```python
from build123d import *

# Parameters (mm, degrees)
SKETCH1_W          = 76
SKETCH1_H          = 76
SKETCH1_R          = 2
SKETCH1_R_2        = 16.65
BASE_FLANGE1_DEPTH = 1.6


# Sheet-metal steps are written as plain solids
with BuildPart() as part:
    # Sketch1 → Base-Flange1 (new body)
    with BuildSketch(Plane(origin=(0, 0, 0), x_dir=(1, 0, 0), z_dir=(0, 1, 0))):
        Rectangle(SKETCH1_W, SKETCH1_H)
        with Locations(Location((32.55, 32.55, 0), (0, 0, 270))):
            Circle(SKETCH1_R, mode=Mode.SUBTRACT)
        with Locations(Location((0, 0, 0), (0, 0, 270))):
            Circle(SKETCH1_R_2, mode=Mode.SUBTRACT)
        with Locations(Location((32.55, -32.55, 0), (0, 0, 270))):
            Circle(SKETCH1_R, mode=Mode.SUBTRACT)
        with Locations(Location((-32.55, -32.55, 0), (0, 0, 270))):
            Circle(SKETCH1_R, mode=Mode.SUBTRACT)
        with Locations(Location((-32.55, 32.55, 0), (0, 0, 270))):
            Circle(SKETCH1_R, mode=Mode.SUBTRACT)
    extrude(amount=-BASE_FLANGE1_DEPTH)


solid = part.part
```
Could you check a few things on this model? Use its own coordinates, in mm. Round coordinates to 2 decimals unless told otherwise and drop trailing zeros. Loops run counter-clockwise (first coordinate to the right, second up) from the corner with the lowest first, then second, coordinate; pieces in that order, holes last. Notation, with made-up numbers: (-28, -17.5) -> (-21, -17.5) arc R24 ccw to (-21, 12.5) -> close; hole circle Ø7 at (58, -9). An arc over 180 degrees is marked (long way). One line per question, with ' | ' between items.
(1) For pin 1 Ø5 at (x, z) = (-32.55, 32.55) entering from +Y; pin 2 Ø3.5 at (x, z) = (32.55, -32.55) entering from -Y, each with a flat end and sliding along its axis, tell me the tip position at first contact or that it passes through.
Model answer:
pin 1: stops at y = 0 | pin 2: passes through
(2) If I drill on probe 1 along X at (y, z) = (-0.35, -32.55); probe 2 along X at (y, z) = (-1.2, 0); probe 3 along X at (y, z) = (-0.95, 14.5), over which ranges is the centre line in solid material (lowest first)?
Model answer:
probe 1: x = -38 to -34.55, -30.55 to 30.55, 34.55 to 38 | probe 2: x = -38 to -16.65, 16.65 to 38 | probe 3: x = -38 to -8.18, 8.18 to 38
(3) If we section it at D-D on y = -0.4: List the corners of the cut face in (x, z) for me.
Model answer:
outline: (-38, -38) -> (38, -38) -> (38, 38) -> (-38, 38) -> close; hole circle Ø4 at (-32.55, -32.55); hole circle Ø4 at (-32.55, 32.55); hole circle Ø33.3 at (0, 0); hole circle Ø4 at (32.55, -32.55); hole circle Ø4 at (32.55, 32.55)
(4) If we section it at C-C on z = 32.55: List the corners of the cut face in (x, y) for me, and give its area (3 significant figures).
Model answer:
outline: (-38, -1.6) -> (-34.55, -1.6) -> (-34.55, 0) -> (-38, 0) -> close; (-30.55, -1.6) -> (30.55, -1.6) -> (30.55, 0) -> (-30.55, 0) -> close; (34.55, -1.6) -> (38, -1.6) -> (38, 0) -> (34.55, 0) -> close | area: 109 mm^2
(5) If we section it at A-A on x = 32.55: List the corners of the cut face in (y, z) for me.
Model answer:
outline: (-1.6, -38) -> (0, -38) -> (0, -34.55) -> (-1.6, -34.55) -> close; (-1.6, -30.55) -> (0, -30.55) -> (0, 30.55) -> (-1.6, 30.55) -> close; (-1.6, 34.55) -> (0, 34.55) -> (0, 38) -> (-1.6, 38) -> close
(6) Thinking about a two-plate mould opening in Z: for faces 1 (the face through (-17, -1.6, -1)), 2 (the face through (-30.567, -0.789, 32.29)), which applies, released by +Z, released by -Z, zero draft, split by the parting line, or undercut?
Model answer:
face 1: zero draft | face 2: undercut
(7) If we section it at B-B on z = 0: List the corners of the cut face in (x, y) for me.
Model answer:
outline: (-38, -1.6) -> (-16.65, -1.6) -> (-16.65, 0) -> (-38, 0) -> close; (16.65, -1.6) -> (38, -1.6) -> (38, 0) -> (16.65, 0) -> close
